```python
from build123d import *

# Parameters (mm, degrees)
F2_R = 5.08


with BuildPart() as f1:
    # F0 (on Front) → F1 (revolve)
    with BuildSketch(Plane.XZ):
        Polygon((23.340716958, 17.2953996807), (-13.42510432, 11.1656589434), (-17.0120093971, -26.6356188804), (0, -28.2498622709), (10.1139964536, -14.769744128), align=None)
    revolve(axis=Axis((-15.2185568586, 0, -7.7349799685), (-0.0944641449, 0, -0.9955282645)))

    # F2
    f2_edges = [f1.edges().sort_by_distance(p)[0] for p in [
        (-34.024019, 0, -25.021375),
        (-41.422124, 0, -9.879561),
        (5.056998, 0, -21.509803),
        (-48.381865, 0, 24.101045),
        (16.727357, 0, 1.262828),
    ]]
    fillet(f2_edges, radius=F2_R)


solid = f1.part
```
Verification items for the finished model (mm, model axes). Round coordinates to 2 decimals unless told otherwise and drop trailing zeros. Answer as a JSON object with one key per item and string values. Group by question number.
Q1. Thickness scan on line 1 (Y direction, x = -10.5, z = -18.5); line 2 (Z direction, x = -18, y = -10.5); line 3 (Y direction, x = 4.5, z = -18). Record the ranges inside material, lowest first.
Q2. Go/stop test with flat-tipped pins: pin 1 Ø2 at (x, y) = (-6.5, -24.5) entering from +Z; pin 2 Ø2 at (y, z) = (2.5, 12.5) entering from -X; pin 3 Ø4 at (x, y) = (-26.5, 11.5) entering from +Z. Record where each tip stops, or that it passes through.
Q3. Mould release check, pull along Y, two halves, no side actions. Record for faces 1 (the conical face through (-12.18, 0.51, 11.4)), 2 (the flat face through (-16.814, -0.199, -26.654)), 3 (the conical face through (1.336, -5.71, -25.221)): released by +Y, released by -Y, zero draft, split by the parting line, or undercut.
Found:
{
 "1": {"line 1": "y = -21.68 to 21.68", "line 2": "z = -26.54 to 14.69", "line 3": "y = -11.5 to 11.5"},
 "2": {"pin 1": "stops at z = 17.52", "pin 2": "stops at x = -46.13", "pin 3": "stops at z = 17.86"},
 "3": {"face 1": "undercut", "face 2": "zero draft", "face 3": "split by the parting line"}
}
